Source: CAD feature listing. Evaluate the final solid. Frame: model axes, mm. Round coordinates to 2 decimals unless told otherwise and drop trailing zeros. Loops run counter-clockwise (first coordinate to the right, second up) from the corner with the lowest first, then second, coordinate; pieces in that order, holes last. Notation, with made-up numbers: M 81,66.5 L 95,66.5 A26 ccw 95,97.5 Z; hole C 42.5,62 d3. An arc over 180 degrees is marked long. Answer as CSV lines item,"result". Start each with the question number.
```python
from build123d import *

# Parameters (mm, degrees)
BOSS_EXTRUDE1_DEPTH                     = 300
CBORE_FOR_M3_PAN_HEAD_SCREW1_AT_2_COUNT = 2
CBORE_FOR_M3_PAN_HEAD_SCREW1_AT_2_PITCH = 20
LPATTERN1_COUNT                         = 13
LPATTERN1_PITCH                         = 20


with BuildPart() as part:
    # Sketch1 → Boss-Extrude1 (new body)
    with BuildSketch(Plane.XY):
        Polygon((-4.005025253, 6.5), (4.005025253, 6.5), (4.5, 6.005025253), (4.5, 5.205025253), (4.005025253, 4.710050506), (3.510050506, 4.710050506), (3.25, 4.45), (3.25, 3.65), (3.510050506, 3.389949494), (4.005025253, 3.389949494), (4.5, 2.894974747), (4.5, 0.494974747), (4.005025253, 0), (-4.005025253, 0), (-4.5, 0.494974747), (-4.5, 2.894974747), (-4.005025253, 3.389949494), (-3.510050506, 3.389949494), (-3.25, 3.65), (-3.25, 4.45), (-3.510050506, 4.710050506), (-4.005025253, 4.710050506), (-4.5, 5.205025253), (-4.5, 6.005025253), align=None)
    extrude(amount=BOSS_EXTRUDE1_DEPTH)

    # Sketch3 → CBORE for M3 Pan Head Screw1 (revolve, cut)
    with BuildSketch(Plane(origin=(0, 6.5, 20), x_dir=(0, 0, 1), z_dir=(1, 0, 0))):
        Polygon((0, 0), (0, 6.5), (1.75, 6.5), (1.75, 3.5), (3, 3.5), (3, 0.25), (3.25, 0), align=None)
    cbore_for_m3_pan_head_screw1 = revolve(axis=Axis((0, 12.85, 20), (0, -1, 0)), mode=Mode.SUBTRACT)

    # CBORE for M3 Pan Head Screw1 at 2: CBORE for M3 Pan Head Screw1 ×2
    with Locations(*[(0, 0, i * CBORE_FOR_M3_PAN_HEAD_SCREW1_AT_2_PITCH) for i in range(1, CBORE_FOR_M3_PAN_HEAD_SCREW1_AT_2_COUNT)]):
        add(cbore_for_m3_pan_head_screw1, mode=Mode.SUBTRACT)

    # LPattern1: CBORE for M3 Pan Head Screw1 ×13
    with Locations(*[(0, 0, i * LPATTERN1_PITCH) for i in range(1, LPATTERN1_COUNT)]):
        add(cbore_for_m3_pan_head_screw1, mode=Mode.SUBTRACT)

    # LPattern1 copy 1 sketch → LPattern1 copy 1 (revolve, cut)
    with BuildSketch(Plane(origin=(0, 6.5, 60), x_dir=(0, 0, 1), z_dir=(1, 0, 0))):
        Polygon((0, 0), (0, 6.5), (1.75, 6.5), (1.75, 3.5), (3, 3.5), (3, 0.25), (3.25, 0), align=None)
    revolve(axis=Axis((0, 12.85, 60), (0, -1, 0)), mode=Mode.SUBTRACT)

    # LPattern1 copy 2 sketch → LPattern1 copy 2 (revolve, cut)
    with BuildSketch(Plane(origin=(0, 6.5, 80), x_dir=(0, 0, 1), z_dir=(1, 0, 0))):
        Polygon((0, 0), (0, 6.5), (1.75, 6.5), (1.75, 3.5), (3, 3.5), (3, 0.25), (3.25, 0), align=None)
    revolve(axis=Axis((0, 12.85, 80), (0, -1, 0)), mode=Mode.SUBTRACT)

    # LPattern1 copy 3 sketch → LPattern1 copy 3 (revolve, cut)
    with BuildSketch(Plane(origin=(0, 6.5, 100), x_dir=(0, 0, 1), z_dir=(1, 0, 0))):
        Polygon((0, 0), (0, 6.5), (1.75, 6.5), (1.75, 3.5), (3, 3.5), (3, 0.25), (3.25, 0), align=None)
    revolve(axis=Axis((0, 12.85, 100), (0, -1, 0)), mode=Mode.SUBTRACT)

    # LPattern1 copy 4 sketch → LPattern1 copy 4 (revolve, cut)
    with BuildSketch(Plane(origin=(0, 6.5, 120), x_dir=(0, 0, 1), z_dir=(1, 0, 0))):
        Polygon((0, 0), (0, 6.5), (1.75, 6.5), (1.75, 3.5), (3, 3.5), (3, 0.25), (3.25, 0), align=None)
    revolve(axis=Axis((0, 12.85, 120), (0, -1, 0)), mode=Mode.SUBTRACT)

    # LPattern1 copy 5 sketch → LPattern1 copy 5 (revolve, cut)
    with BuildSketch(Plane(origin=(0, 6.5, 140), x_dir=(0, 0, 1), z_dir=(1, 0, 0))):
        Polygon((0, 0), (0, 6.5), (1.75, 6.5), (1.75, 3.5), (3, 3.5), (3, 0.25), (3.25, 0), align=None)
    revolve(axis=Axis((0, 12.85, 140), (0, -1, 0)), mode=Mode.SUBTRACT)

    # LPattern1 copy 6 sketch → LPattern1 copy 6 (revolve, cut)
    with BuildSketch(Plane(origin=(0, 6.5, 160), x_dir=(0, 0, 1), z_dir=(1, 0, 0))):
        Polygon((0, 0), (0, 6.5), (1.75, 6.5), (1.75, 3.5), (3, 3.5), (3, 0.25), (3.25, 0), align=None)
    revolve(axis=Axis((0, 12.85, 160), (0, -1, 0)), mode=Mode.SUBTRACT)

    # LPattern1 copy 7 sketch → LPattern1 copy 7 (revolve, cut)
    with BuildSketch(Plane(origin=(0, 6.5, 180), x_dir=(0, 0, 1), z_dir=(1, 0, 0))):
        Polygon((0, 0), (0, 6.5), (1.75, 6.5), (1.75, 3.5), (3, 3.5), (3, 0.25), (3.25, 0), align=None)
    revolve(axis=Axis((0, 12.85, 180), (0, -1, 0)), mode=Mode.SUBTRACT)

    # LPattern1 copy 8 sketch → LPattern1 copy 8 (revolve, cut)
    with BuildSketch(Plane(origin=(0, 6.5, 200), x_dir=(0, 0, 1), z_dir=(1, 0, 0))):
        Polygon((0, 0), (0, 6.5), (1.75, 6.5), (1.75, 3.5), (3, 3.5), (3, 0.25), (3.25, 0), align=None)
    revolve(axis=Axis((0, 12.85, 200), (0, -1, 0)), mode=Mode.SUBTRACT)

    # LPattern1 copy 9 sketch → LPattern1 copy 9 (revolve, cut)
    with BuildSketch(Plane(origin=(0, 6.5, 220), x_dir=(0, 0, 1), z_dir=(1, 0, 0))):
        Polygon((0, 0), (0, 6.5), (1.75, 6.5), (1.75, 3.5), (3, 3.5), (3, 0.25), (3.25, 0), align=None)
    revolve(axis=Axis((0, 12.85, 220), (0, -1, 0)), mode=Mode.SUBTRACT)

    # LPattern1 copy 10 sketch → LPattern1 copy 10 (revolve, cut)
    with BuildSketch(Plane(origin=(0, 6.5, 240), x_dir=(0, 0, 1), z_dir=(1, 0, 0))):
        Polygon((0, 0), (0, 6.5), (1.75, 6.5), (1.75, 3.5), (3, 3.5), (3, 0.25), (3.25, 0), align=None)
    revolve(axis=Axis((0, 12.85, 240), (0, -1, 0)), mode=Mode.SUBTRACT)

    # LPattern1 copy 11 sketch → LPattern1 copy 11 (revolve, cut)
    with BuildSketch(Plane(origin=(0, 6.5, 260), x_dir=(0, 0, 1), z_dir=(1, 0, 0))):
        Polygon((0, 0), (0, 6.5), (1.75, 6.5), (1.75, 3.5), (3, 3.5), (3, 0.25), (3.25, 0), align=None)
    revolve(axis=Axis((0, 12.85, 260), (0, -1, 0)), mode=Mode.SUBTRACT)

    # LPattern1 copy 12 sketch → LPattern1 copy 12 (revolve, cut)
    with BuildSketch(Plane(origin=(0, 6.5, 280), x_dir=(0, 0, 1), z_dir=(1, 0, 0))):
        Polygon((0, 0), (0, 6.5), (1.75, 6.5), (1.75, 3.5), (3, 3.5), (3, 0.25), (3.25, 0), align=None)
    revolve(axis=Axis((0, 12.85, 280), (0, -1, 0)), mode=Mode.SUBTRACT)


solid = part.part
```
1) Section A-A, the plane z = 206. Return loops of the section in (x, y).
2) Mould query, pull axis Z, two halves, no side actions, for faces 1 (the flat face through (0, 3, 0)), 2 (the flat face through (0, 3, 300)), 3 (the flat face through (0, 3, 278)). Classes: pulls with the +Z half, pulls with the -Z half, needs draft (parallel to the pull), parting line crosses it, or undercut.
3) Ray query, line 1 along X through (y, z) = (1.6, 280); line 2 along Y through (x, z) = (-3.5, 207); line 3 along X through (y, z) = (4.25, 40). Return the intervals inside material, ascending.
4) Contact query for flat-ended pins moving along their axis: pin 1 Ø1.8 at (x, z) = (-1, 140.5) entering from +Y; pin 2 Ø3 at (x, z) = (0, 180) entering from +Y. Output: stop coordinate, or through.
5) Section B-B, the plane x = 0. Give the number of separate pieces and of enclosed holes in the cut face, and give its area (3 significant figures).
Findings below:
1,outline,"M -4.5,0.49 L -4.01,0 L 4.01,0 L 4.5,0.49 L 4.5,2.89 L 4.01,3.39 L 3.51,3.39 L 3.25,3.65 L 3.25,4.45 L 3.51,4.71 L 4.01,4.71 L 4.5,5.21 L 4.5,6.01 L 4.01,6.5 L -4.01,6.5 L -4.5,6.01 L -4.5,5.21 L -4.01,4.71 L -3.51,4.71 L -3.25,4.45 L -3.25,3.65 L -3.51,3.39 L -4.01,3.39 L -4.5,2.89 Z"
2,face 1,"pulls with the -Z half"
2,face 2,"pulls with the +Z half"
2,face 3,"undercut"
3,line 1,"-4.5 to -1.75, 1.75 to 4.5"
3,line 2,"0 to 3.4, 4.7 to 6.5"
3,line 3,"-3.25 to -3, 3 to 3.25"
4,pin 1,"y = 3"
4,pin 2,"through"
5,separate pieces,"15"
5,enclosed holes,"0"
5,area,"1,510 mm²"
